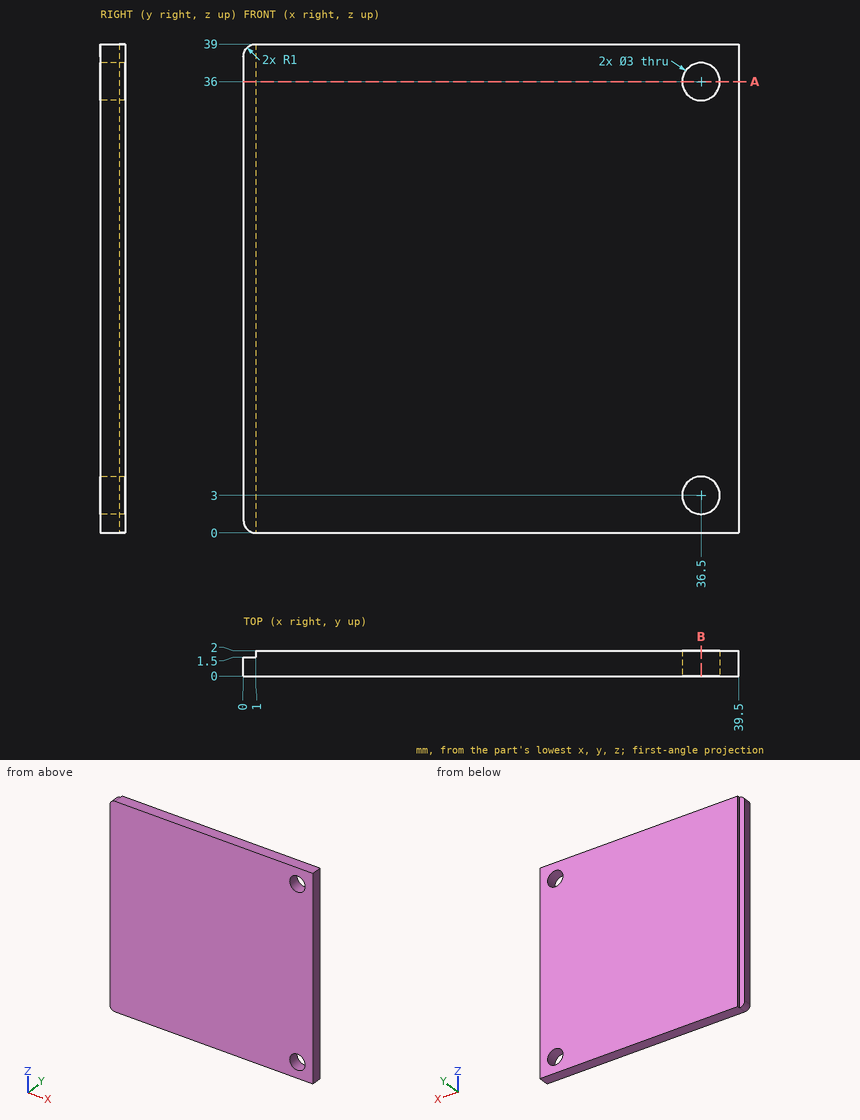
Verification items for this drawing (mm, ordinates from the low corner). Coordinates: 2 decimals unless noted, no trailing zeros. Loops run counter-clockwise (first coordinate to the right, second up) from the corner with the lowest first, then second, coordinate; pieces in that order, holes last. Notation, with made-up numbers: (78.25, 82) -> (101.25, 82) arc R25 cw to (101.25, 119) -> close; hole circle Ø11 at (74, 77). An arc over 180 degrees is marked (long way). Answer in a Markdown table with one row per item. Add a question column.
1. Material ranges on probe 1 along Z at (x, y) = (36.5, 0.6); probe 2 along X at (y, z) = (1.2, 36); probe 3 along X at (y, z) = (0.4, 36.5), recorded low to high. Write a range as [from, to].
2. Section check B-B, the plane x = 36.5. Enter the section's corners in (y, z), then the cut area to 3 significant figures.
3. Section check A-A, the plane z = 36. Enter the section's corners in (x, y), then the cut area to 3 significant figures.
4. Depth check by flat-ended pin: P1, Ø0.6, axis at y = 2, z = 14.5, coming from the -X side. Enter the tip coordinate at first touch or a pass-through.
Derived:
| question | item | result |
|---|---|---|
| 1 | probe 1 | z = [0, 1.5], [4.5, 34.5], [37.5, 39] |
| 1 | probe 2 | x = [0, 35], [38, 39.5] |
| 1 | probe 3 | x = [0, 35.09], [37.91, 39.5] |
| 2 | outline | (0, 0) -> (2, 0) -> (2, 1.5) -> (0, 1.5) -> close; (0, 4.5) -> (2, 4.5) -> (2, 34.5) -> (0, 34.5) -> close; (0, 37.5) -> (2, 37.5) -> (2, 39) -> (0, 39) -> close |
| 2 | area | 66.0 mm² |
| 3 | outline | (0, 0) -> (35, 0) -> (35, 2) -> (1, 2) -> (1, 1.5) -> (0, 1.5) -> close; (38, 0) -> (39.5, 0) -> (39.5, 2) -> (38, 2) -> close |
| 3 | area | 72.5 mm² |
| 4 | P1 | stops at x = 1 |
